Design review of the part built by this model. Coordinates are the model's own, in mm. Face numbers are marked on the shaded views. A direction names the side the tool comes from. Round coordinates to 2 decimals unless told otherwise and drop trailing zeros. Loops run counter-clockwise (first coordinate to the right, second up) from the corner with the lowest first, then second, coordinate; pieces in that order, holes last. Notation, with made-up numbers: (81.25, 46) - (129.25, 46) arc R25 ccw to (129.25, 60) - close; hole circle Ø1 at (59.5, 78). An arc over 180 degrees is marked (long way). Answer as CSV lines item,"result". Start each with the question number.
(1) Mouldability with a two-part tool opening along Y and no side actions: class the marked faces 4, 5, 6 and 7 as released by +Y, released by -Y, zero draft, split by the parting line, or undercut.
(2) Consider section C-C (x = 57). Give the boundary of the cut face in (y, z).
(3) For the marked faces 1, 2 and 3, list the 3-axis set-ups (+Z, -Z, +X, -X, +Y, -Y) from which the entire face can be reached by the end or side of a thin tool; tool diameter is ignored.
(4) Wall thickness on L1, parallel to Y at x = 94, z = 46.5; L2, parallel to X at y = 6.25, z = 30; L3, parallel to X at y = 50, z = 129.5: over which ranges is each line inside the solid? List them lowest first.
(5) For P1, Ø8, axis at y = 47.5, z = 16.5, coming from the +X side; P2, Ø10, axis at x = 63.5, y = 62, coming from the +Z side; P3, Ø5, axis at y = 31, z = 35, coming from the -X side, all flat-tipped, find the tip position at first contact; note any pin that passes through.
(6) Consider section A-A (x = 37). Give the boundary of the cut face in (y, z).
(7) Consider section D-D (z = 93.5). Give the boundary of the cut face in (x, y), and give its area (3 significant figures).
(8) Consider section B-B (z = 123). Give the boundary of the cut face in (x, y).
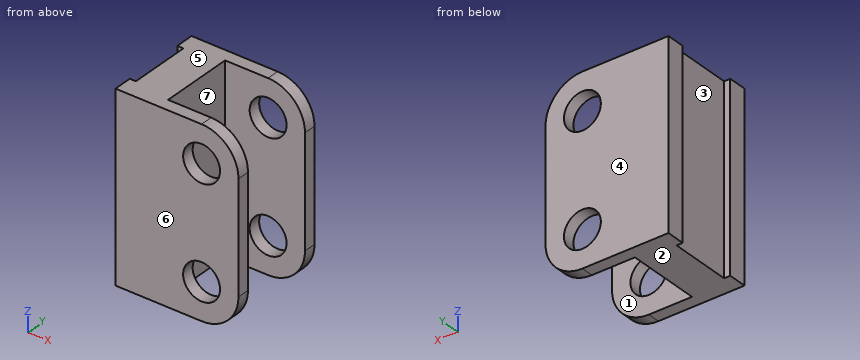
from build123d import *

# Parameters (mm, degrees)
BOSS_EXTRUDE1_DEPTH = 150
SKETCH2_W           = 5
SKETCH2_H           = 50
CUT_EXTRUDE1_DEPTH  = 150
SKETCH3_R           = 15
CUT_EXTRUDE2_DEPTH  = 150
FILLET1_R           = 30


with BuildPart() as part:
    # Sketch1 → Boss-Extrude1 (new body)
    with BuildSketch(Plane.XY):
        Polygon((0, 0), (35, 0), (100, 0), (100, 10), (35, 10), (35, 70), (100, 70), (100, 80), (35, 80), (0, 80), align=None)
    extrude(amount=BOSS_EXTRUDE1_DEPTH)

    # Sketch2 → Cut-Extrude1 (cut)
    with BuildSketch(Plane.XY.offset(150)):
        with Locations((2.5, 40)):
            Rectangle(SKETCH2_W, SKETCH2_H)
    extrude(amount=-CUT_EXTRUDE1_DEPTH, mode=Mode.SUBTRACT)

    # Sketch3 → Cut-Extrude2 (cut)
    with BuildSketch(Plane(origin=(0, 80, 0), x_dir=(1, 0, 0), z_dir=(0, 1, 0))):
        with Locations(Location((70, -30, 0), (0, 0, 270))):
            Circle(SKETCH3_R)
        with Locations(Location((70, -120, 0), (0, 0, 270))):
            Circle(SKETCH3_R)
    extrude(amount=-CUT_EXTRUDE2_DEPTH, mode=Mode.SUBTRACT)

    # Fillet1
    fillet1_edges = [part.edges().sort_by_distance(p)[0] for p in [
        (100, 75, 0),
        (100, 5, 0),
        (100, 5, 150),
        (100, 75, 150),
    ]]
    fillet(fillet1_edges, radius=FILLET1_R)


solid = part.part
Determined:
1,face 4,"released by +Y"
1,face 5,"zero draft"
1,face 6,"released by -Y"
1,face 7,"undercut"
2,outline,"(0, 0) - (10, 0) - (10, 22.52) - (0, 22.52) - close; (0, 37.48) - (10, 37.48) - (10, 112.52) - (0, 112.52) - close; (0, 127.48) - (10, 127.48) - (10, 150) - (0, 150) - close; (70, 0) - (80, 0) - (80, 22.52) - (70, 22.52) - close; (70, 37.48) - (80, 37.48) - (80, 112.52) - (70, 112.52) - close; (70, 127.48) - (80, 127.48) - (80, 150) - (70, 150) - close"
3,face 1,"+Z, -Z, +X"
3,face 2,"-Z, +X, -X, +Y, -Y"
3,face 3,"+Z, -Z, -X"
4,L1,"y = 0 to 10, 70 to 80"
4,L2,"x = 0 to 55, 85 to 100"
4,L3,"x = 5 to 35"
5,P1,"stops at x = 35"
5,P2,"passes through"
5,P3,"stops at x = 5"
6,outline,"(0, 0) - (10, 0) - (10, 150) - (0, 150) - close; (70, 0) - (80, 0) - (80, 150) - (70, 150) - close"
7,outline,"(0, 0) - (100, 0) - (100, 10) - (35, 10) - (35, 70) - (100, 70) - (100, 80) - (0, 80) - (0, 65) - (5, 65) - (5, 15) - (0, 15) - close"
7,area,"3,850 mm^2"
8,outline,"(0, 0) - (55.3, 0) - (55.3, 10) - (35, 10) - (35, 70) - (55.3, 70) - (55.3, 80) - (0, 80) - (0, 65) - (5, 65) - (5, 15) - (0, 15) - close; (84.7, 0) - (99.85, 0) - (99.85, 10) - (84.7, 10) - close; (84.7, 70) - (99.85, 70) - (99.85, 80) - (84.7, 80) - close"
